Design review of the part built by this model. Coordinates are the model's own, in mm. A direction names the side the tool comes from. Give positions to 0.01 mm unless a question says otherwise; leave off trailing zeros. Write each loop counter-clockwise with the first axis right and the second up, starting at its lowest first coordinate (ties: lowest second). Pieces come first, ordered by that corner, then holes. Notation, with made-up numbers: M 8.25,62 L 33.25,62 A32 ccw 33.25,90 Z; hole C 40.5,27 d4. An arc over 180 degrees is marked long. Answer in a Markdown table with one row per item.
```python
from build123d import *

# Parameters (mm, degrees)
SKETCH3_W   = 914.4
SKETCH3_H   = 609.6
TABLE_DEPTH = 25.4
SKETCH4_R   = 19.05
LEGS_DEPTH  = 794.675


with BuildPart() as part:
    # Sketch3 → Table (new body)
    with BuildSketch(Plane(origin=(0, 0, 0), x_dir=(1, 0, 0), z_dir=(0, 1, 0))):
        with Locations((457.2, 304.8)):
            Rectangle(SKETCH3_W, SKETCH3_H)
    extrude(amount=TABLE_DEPTH)

    # Sketch4 → Legs (add)
    with BuildSketch(Plane.XZ):
        with Locations((50.8, -50.8)):
            Circle(SKETCH4_R)
        with Locations((863.6, -50.8)):
            Circle(SKETCH4_R)
        with Locations((50.8, -558.8)):
            Circle(SKETCH4_R)
        with Locations((863.6, -558.8)):
            Circle(SKETCH4_R)
    extrude(amount=LEGS_DEPTH)


solid = part.part
```
1) Add section C-C (y = -61). Write out the cut boundary in (x, z), and give its area (3 significant figures).
Geometry says:
| item | result |
|---|---|
| outline | C 50.8,-558.8 d38.1; C 50.8,-50.8 d38.1; C 863.6,-558.8 d38.1; C 863.6,-50.8 d38.1 |
| area | 4,560 mm^2 |
2) Add section B-B (z = -558.8). Write out the cut boundary in (x, y) (3 decimals), and give its area (3 significant figures).
Geometry says:
| item | result |
|---|---|
| outline | M 0,0 L 31.75,0 L 31.75,-794.675 L 69.85,-794.675 L 69.85,0 L 844.55,0 L 844.55,-794.675 L 882.65,-794.675 L 882.65,0 L 914.4,0 L 914.4,25.4 L 0,25.4 Z |
| area | 83,800 mm^2 |
3) For faces 1 (the face through (0, 13, -301)), 2 (the face through (48.32, -391.775, -539.912)), list the 3-axis set-ups (+Z, -Z, +X, -X, +Y, -Y) from which the entire face can be reached by the end or side of a thin tool; tool diameter is ignored.
Geometry says:
| item | result |
|---|---|
| face 1 | +Z, -Z, -X, +Y, -Y |
| face 2 | -Y |
4) To check wall thickness, follow probe 1 along Y at (x, z) = (541.5, -386); probe 2 along Z at (x, y) = (63.5, -683.5); probe 3 along X at (y, z) = (-84, -66). State the ranges of each line that lie inside material, in increasing order. Write a range as [from, to].
Geometry says:
| item | result |
|---|---|
| probe 1 | [0, 25.4] |
| probe 2 | [-573, -544.6], [-65, -36.6] |
| probe 3 | [39.32, 62.28], [852.12, 875.08] |
5) Add section D-D (z = -331). Write out the cut boundary in (x, y).
Geometry says:
| item | result |
|---|---|
| outline | M 0,0 L 914.4,0 L 914.4,25.4 L 0,25.4 Z |
6) Add section A-A (x = 50.8). Write out the cut boundary in (y, z) (3 decimals).
Geometry says:
| item | result |
|---|---|
| outline | M -794.675,-577.85 L 0,-577.85 L 0,-609.6 L 25.4,-609.6 L 25.4,0 L 0,0 L 0,-31.75 L -794.675,-31.75 L -794.675,-69.85 L 0,-69.85 L 0,-539.75 L -794.675,-539.75 Z |
